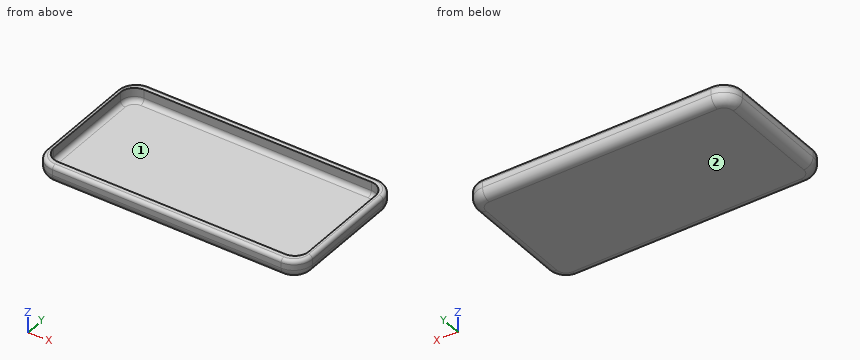
from build123d import *

# Parameters (mm, degrees)
F0_W     = 144
F0_H     = 72
F1_DEPTH = 10
F3_DEPTH = 3
F2_W     = 138.3
F2_H     = 67.1
F4_DEPTH = 7.2
F5_R     = 7.5
F6_R     = 2.5
F7_R     = 10
F8_R     = 2
F9_R     = 5


with BuildPart() as f1:
    # F0 (on Top) → F1 (new body)
    with BuildSketch(Plane.XY):
        with Locations((-65.7520391978, -7.4041044508)):
            Rectangle(F0_W, F0_H)
    extrude(amount=F1_DEPTH)

    # F3 (add): a face of the model
    f3_faces = [f1.faces().sort_by_distance(p)[0] for p in [
        (-65.7520391978, 28.5958955492, 5),
    ]]
    extrude(f3_faces, amount=F3_DEPTH)

    # F2 (on face) → F4 (cut)
    with BuildSketch(Plane.XY.offset(10)):
        with Locations((-66.0260241712, -5.8019728968)):
            Rectangle(F2_W, F2_H)
    extrude(amount=-F4_DEPTH, mode=Mode.SUBTRACT)

    # F5
    f5_edges = [f1.edges().sort_by_distance(p)[0] for p in [
        (-135.176024, 27.748027, 6.4),
        (-135.176024, -39.351973, 6.4),
        (3.123976, -39.351973, 6.4),
        (3.123976, 27.748027, 6.4),
    ]]
    fillet(f5_edges, radius=F5_R)

    # F6
    f6_edges = [f1.edges().sort_by_distance(p)[0] for p in [
        (-66.026024, 27.748027, 2.8),
    ]]
    fillet(f6_edges, radius=F6_R)

    # F7
    f7_edges = [f1.edges().sort_by_distance(p)[0] for p in [
        (-137.752039, -43.404104, 5),
        (6.247961, -43.404104, 5),
        (6.247961, 31.595896, 5),
        (-137.752039, 31.595896, 5),
    ]]
    fillet(f7_edges, radius=F7_R)

    # F8
    f8_edges = [f1.edges().sort_by_distance(p)[0] for p in [
        (-65.752039, -43.404104, 10),
        (-65.752039, 31.595896, 10),
        (-137.752039, -5.904104, 10),
    ]]
    fillet(f8_edges, radius=F8_R)

    # F9
    f9_edges = [f1.edges().sort_by_distance(p)[0] for p in [
        (-65.752039, -43.404104, 0),
        (-134.823107, -40.475172, 0),
        (3.319029, -40.475172, 0),
        (-137.752039, -5.904104, 0),
        (6.247961, -5.904104, 0),
        (-134.823107, 28.666963, 0),
        (3.319029, 28.666963, 0),
        (-65.752039, 31.595896, 0),
    ]]
    fillet(f9_edges, radius=F9_R)


solid = f1.part
Can you work these out from the model? Positions are in its coordinate system, mm. Face numbers are marked on the shaded views. Coordinates: 2 decimals unless noted, no trailing zeros. Order: outer loops, then holes, each group sorted by start corner. A loop starts at its lowest first (then second) coordinate and runs counter-clockwise, first axis right, second up. Notation, with made-up numbers: (-15, -36.5) - (44, -36.5) arc R23 cw to (44, -10.5) - close; hole circle Ø9 at (39, 78). An arc over 180 degrees is marked (long way). Answer as a JSON object with one key per item and string values. Group by question number.
Q1. I need wall thicknesses on line 1 (Y direction, x = -14.5, z = 5.5); line 2 (Y direction, x = -19, z = 5); line 3 (X direction, y = -4, z = 6.5). Which ranges of each line are inside material? Lowest first, please. Write a range as from..to.
Q2. We'd pull the mould along Y, two halves only. Please class the marked faces 1 and 2: +Y half, -Y half, draft (parallel to the pull), parting line (faces both ways), or undercut.
Q3. Will this pin go through, and if not, where does the flat tip stop? P1, Ø10, axis at x = -66.5, y = -19.5, coming from the +Z side.
Q4. Imagine slicing it at A-A (y = -1.5). Please give me the cut outline in (x, z), and give its area (3 significant figures).
Q5. Imagine slicing it at B-B (x = -116.5). Please give me the cut outline in (y, z).
Determined:
{
 "1": {"line 1": "y = -43.4..-39.35, 27.75..31.6", "line 2": "y = -43.4..-39.33, 27.73..31.6", "line 3": "x = -137.75..-135.18, 3.12..6.25"},
 "2": {"face 1": "undercut", "face 2": "draft"},
 "3": {"P1": "stops at z = 2.8"},
 "4": {"outline": "(-137.75, 5) arc R5 ccw to (-132.75, 0) - (1.25, 0) arc R5 ccw to (6.25, 5) - (6.25, 8) arc R2 ccw to (4.25, 10) - (3.12, 10) - (3.12, 5.3) arc R2.5 cw to (0.62, 2.8) - (-132.68, 2.8) arc R2.5 cw to (-135.18, 5.3) - (-135.18, 10) - (-135.75, 10) arc R2 ccw to (-137.75, 8) - close", "area": "434 mm2"},
 "5": {"outline": "(-43.4, 5) arc R5 ccw to (-38.4, 0) - (26.6, 0) arc R5 ccw to (31.6, 5) - (31.6, 8) arc R2 ccw to (29.6, 10) - (27.75, 10) - (27.75, 5.3) arc R2.5 cw to (25.25, 2.8) - (-36.85, 2.8) arc R2.5 cw to (-39.35, 5.3) - (-39.35, 10) - (-41.4, 10) arc R2 ccw to (-43.4, 8) - close"}
}
